Drawing for the job (mm, zero at the part's lowest x, y, z). Give positions to 0.01 mm unless a question says otherwise; leave off trailing zeros. Order: outer loops, then holes, each group sorted by start corner. A loop starts at its lowest first (then second) coordinate and runs counter-clockwise, first axis right, second up. Notation, with made-up numbers: (33, 38) -> (45, 38) arc R38 cw to (45, 77) -> close; hole circle Ø1 at (59, 3). An arc over 180 degrees is marked (long way). Use one line per item in the form item = value. Start each with the question number.
1) Drop flat-ended pins along their axis: P1, Ø1, axis at x = 6.5, y = 11.5, coming from the +Z side; P2, Ø5, axis at x = 15.5, z = 19, coming from the +Y side. Give the stop position or say it passes through.
2) Cut at C-C, the plane z = 13. Give the cut face in (x, y), and give its area (3 significant figures).
3) Mould opens along X. For the marked faces 1, 2 and 3 say: pulls with the +X half, pulls with the -X half, needs draft (parallel to the pull), parting line crosses it, or undercut.
4) Cut at A-A, the plane y = 18.25. Give the cut face in (x, z).
5) Cut at D-D, the plane x = 5.5. Give the cut face in (y, z), and give its area (3 significant figures).
6) Cut at B-B, the plane z = 21. Give the cut face in (x, y).
7) Probe line 1 (X direction, y = 21.25, z = 6.75); line 2 (Z direction, x = 19, y = 12.25) (1 decimal); line 3 (Z direction, x = 13, y = 15.75) (1 decimal). List the from-to ranges inside material, lowest first.
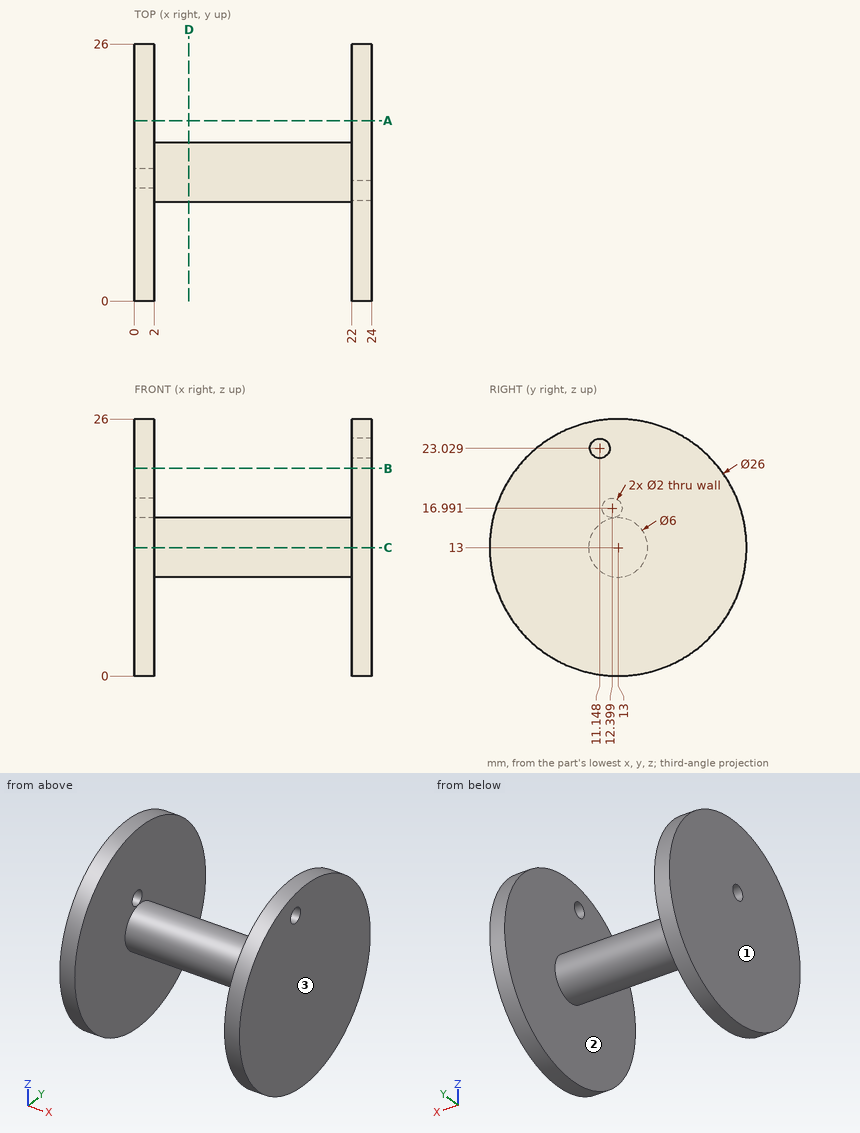
Result:
q1.P1 = 15.83
q1.P2 = through
q2.outline = (0, 0) -> (2, 0) -> (2, 10) -> (22, 10) -> (22, 0) -> (24, 0) -> (24, 26) -> (22, 26) -> (22, 16) -> (2, 16) -> (2, 26) -> (0, 26) -> close
q2.area = 224 mm²
q3.face_1 = pulls with the -X half
q3.face_2 = undercut
q3.face_3 = pulls with the +X half
q4.outline = (0, 1.11) -> (2, 1.11) -> (2, 24.89) -> (0, 24.89) -> close; (22, 1.11) -> (24, 1.11) -> (24, 24.89) -> (22, 24.89) -> close
q5.outline = circle Ø6 at (13, 13)
q5.area = 28.3 mm²
q6.outline = (0, 2.75) -> (2, 2.75) -> (2, 23.25) -> (0, 23.25) -> close; (22, 2.75) -> (24, 2.75) -> (24, 23.25) -> (22, 23.25) -> close
q7.line_1 = 0 to 2, 22 to 24
q7.line_2 = 10.1 to 15.9
q7.line_3 = 11.8 to 14.2
